```python
from build123d import *

# Parameters (mm, degrees)
BOSS_EXTRUDE1_DEPTH = 4.8
CUT_EXTRUDE1_REACH  = 4
SKETCH2_R           = 1.1
CUT_EXTRUDE2_REACH  = 4
SKETCH3_R           = 1.5


with BuildPart() as part:
    # Sketch1 → Boss-Extrude1 (new body)
    with BuildSketch(Plane.XY):
        Polygon((0, 0), (0, 11.8), (-2, 11.8), (-2, 2), (-10, 2), (-10, 0), align=None)
    extrude(amount=BOSS_EXTRUDE1_DEPTH)

    # Sketch2 → Cut-Extrude1 (cut, up to next)
    with BuildSketch(Plane.ZY.offset(2), mode=Mode.PRIVATE) as cut_extrude1_sk1:
        with Locations((2.7, 5.9)):
            Circle(SKETCH2_R)
    cut_extrude1_tool1 = extrude(cut_extrude1_sk1.sketch, amount=-CUT_EXTRUDE1_REACH, mode=Mode.PRIVATE) & part.part
    add(cut_extrude1_tool1.solids().sort_by_distance((-2, 5.9, 2.7))[0], mode=Mode.SUBTRACT)

    # Sketch3 → Cut-Extrude2 (cut, up to next)
    with BuildSketch(Plane(origin=(0, 2, 0), x_dir=(1, 0, 0), z_dir=(0, 1, 0)), mode=Mode.PRIVATE) as cut_extrude2_sk1:
        with Locations((-5.786663097, -2.4)):
            Circle(SKETCH3_R)
    cut_extrude2_tool1 = extrude(cut_extrude2_sk1.sketch, amount=-CUT_EXTRUDE2_REACH, mode=Mode.PRIVATE) & part.part
    add(cut_extrude2_tool1.solids().sort_by_distance((-5.786663, 2, 2.4))[0], mode=Mode.SUBTRACT)


solid = part.part
```
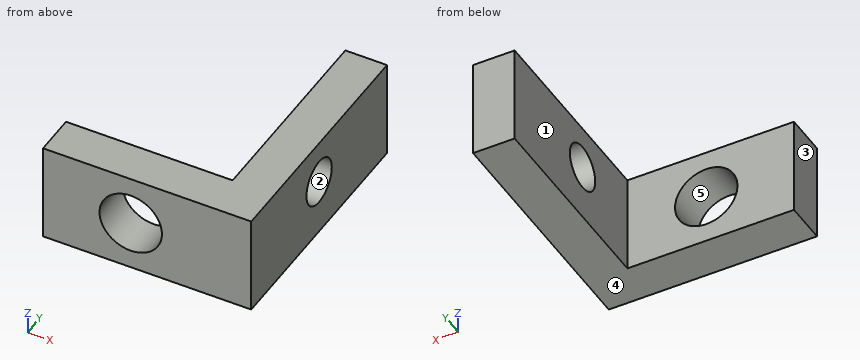
Model file for the job. Use its own axes, mm. Face numbers are marked on the shaded views. A direction names the side the tool comes from. Coordinates: 2 decimals unless noted, no trailing zeros. Write each loop counter-clockwise with the first axis right and the second up, starting at its lowest first coordinate (ties: lowest second). Pieces come first, ordered by that corner, then holes. Notation, with made-up numbers: (-29.5, 88) - (20.5, 88) arc R20 cw to (20.5, 122) - close; hole circle Ø4 at (2, 34). An arc over 180 degrees is marked (long way). Use a Markdown table: item, result. Add a question column.
Item 1: Band-saw the part on C-C, the plane z = 2.4. Write the cut outline in (x, y), and give its area (3 significant figures).
Item 2: Two-plate mould, pull along Z, no slides. Class the marked faces 3, 4 and 5: pulls with the +Z half, pulls with the -Z half, needs draft (parallel to the pull), parting line crosses it, or undercut.
Item 3: 3-axis set-ups, long thin cutter, end or side, ignore diameter. For the marked faces 1 and 2: which of +Z, -Z, +X, -X, +Y, -Y reach the whole face in a straight line?
Item 4: Drop a flat-ended pin along its axis: pin 1 (2.5 mm diameter, centred on x = -5.79, z = 2.4, fed in from +Y). Give the stop position or say it passes through.
Item 5: Band-saw the part on A-A, the plane y = 5.9. Write the cut outline in (x, z).
Item 6: Band-saw the part on D-D, the plane x = -4.5. Write the cut outline in (y, z), and give its area (3 significant figures).
Item 7: Drill centre lines: line 1 along Y through (x, z) = (-1.3, 2.7); line 2 along Y through (x, z) = (-3, 2.9); line 3 along X through (y, z) = (3.25, 1.8). Where is each one in solid material? Low to high.
Item 8: Band-saw the part on B-B, the plane z = 1.4. Write the cut outline in (x, y).
A:
| question | item | result |
|---|---|---|
| 1 | outline | (-10, 0) - (-7.29, 0) - (-7.29, 2) - (-10, 2) - close; (-4.29, 0) - (0, 0) - (0, 4.84) - (-2, 4.84) - (-2, 2) - (-4.29, 2) - close; (-2, 6.96) - (0, 6.96) - (0, 11.8) - (-2, 11.8) - close |
| 1 | area | 29.4 mm² |
| 2 | face 3 | needs draft |
| 2 | face 4 | pulls with the -Z half |
| 2 | face 5 | undercut |
| 3 | face 1 | +Z, -Z, -X, +Y |
| 3 | face 2 | +X, -X |
| 4 | pin 1 | passes through |
| 5 | outline | (-2, 0) - (0, 0) - (0, 1.6) - (-2, 1.6) - close; (-2, 3.8) - (0, 3.8) - (0, 4.8) - (-2, 4.8) - close |
| 6 | outline | (0, 0) - (2, 0) - (2, 1.63) - (0, 1.63) - close; (0, 3.17) - (2, 3.17) - (2, 4.8) - (0, 4.8) - close |
| 6 | area | 6.52 mm² |
| 7 | line 1 | y = 0 to 4.8, 7 to 11.8 |
| 7 | line 2 | y = 0 to 2 |
| 7 | line 3 | x = -2 to 0 |
| 8 | outline | (-10, 0) - (-6.9, 0) - (-6.9, 2) - (-10, 2) - close; (-4.67, 0) - (0, 0) - (0, 11.8) - (-2, 11.8) - (-2, 2) - (-4.67, 2) - close |
